Autodesk Inventor part; units mm, degrees
ref_plane "Work Plane1" through (30, 0, 0) normal (0, -0.5, 0.866) x (1, 0, 0)
ref_plane "YZ Plane" through (0, 0, 0) normal (1, 0, 0) x (0, 1, 0)
ref_plane "XZ Plane" through (0, 0, 0) normal (0, 1, 0) x (-1, 0, 0)
sketch "Sketch1" plane through (0, 0, 0) normal (0, 0, 1) x (1, 0, 0)
  line L0 (0.1133, 0) -> (16, 0)
  line L1 (16, 0) -> (16, 3)
  line L2 (16, 3) -> (2, 3)
  line L3 (2, 3) -> (1.3865, 3)
  line L4 (1.3865, 3) -> (0, 3)
  line L5 (0, 3) -> (0, 5.25)
  line L6 (0, 5.25) -> (-3.3, 5.25)
  line L7 (-3.3, 5.25) -> (-3.3, 2.3094)
  line L8 (-3.3, 2.3094) -> (-1.22, 2.3094)
  line L9 (-1.22, 2.3094) -> (0.1133, 0)
  line L10 (-7.16, 0) -> (19.86, 0)
  line L11 (0, -1.05) -> (0, 6.3)
  line L12 (2, 3) -> (0, 3) construction
  dimension "d0" = 14
  dimension "d1" = 0.6135
  dimension "d2" = 3.3
  dimension "d3" = 2.08
  dimension "d4" = 60
  dimension "d5" = 6
  dimension "d6" = 6
  dimension "d7" = 4.6188
  dimension "d8" = 10.5
  dimension "d19" = 16
revolve "Body" add sketch "Sketch1" angle 360 about axis through (0.1133, 0, 0) along (1, 0, 0) contours L9 L11 L4 L3 L2 L1 L0 | L9 L8 L7 L6 L5 L11
sketch "Sketch2" plane through (-3.3, 0, 0) normal (-1, 0, 0) x (0, 0, 1)
  circle A0 centre (0, 0) radius 2.3094
  line L0 (0, -7.35) -> (0, 7.35)
  line L1 (-7.35, 0) -> (7.35, 0)
  line L2 (2.3094, 0) -> (1.1547, -2)
  line L3 (1.1547, -2) -> (-1.1547, -2)
  line L4 (-1.1547, -2) -> (-2.3094, 0)
  line L5 (-2.3094, 0) -> (-1.1547, 2)
  line L6 (-1.1547, 2) -> (1.1547, 2)
  line L7 (1.1547, 2) -> (2.3094, 0)
extrude "Slot" add sketch "Sketch2" against normal up to next contours L7 A0 | A0 L2 | L6 L0 A0 | A0 L0 L3 | L0 L6 A0 | A0 L3 L0 | L4 A0 | A0 L5
fillet "Fillet1" radius 2.5 1 edges at (-3.3, -5.25, 0)
thread "Thread"
chamfer "Chamfer1" distance 0.6135 distance2 0.6135 1 edges at (16, -3, 0) measured on face at (16, -1.1424, 0.935)
fillet "Fillet2" radius 0.25 1 edges at (0, -3, 0)
ref_plane "Work Plane1" through (30, 0, 0) normal (0, -0.5, 0.866) x (1, 0, 0)
equation "\"d0\" = GEL"
equation "\"d1\" = GAL"
equation "\"d2\" = KOH"
equation "\"d3\" = INTI"
equation "\"d5\" = GD"
equation "\"d6\" = BDM"
equation "\"d7\" = 1.1547 * SW"
equation "\"d8\" = KOD"
equation "\"d19\" = NLG"
equation "\"d16\" = RR"
equation "\"d12\" = GEL"
equation "\"d14\" = -0.5 * SPD + 0.5 * GD"
equation "\"d15\" = GUL"
equation "\"d29\" = R"
equation "\"GD\" = NND"
equation "\"NLG\" = 16"
equation "\"GEL\" = 14"
equation "\"KOD\" = 10.5"
equation "\"KOH\" = 3.3"
equation "\"INTI\" = 2.08"
equation "\"GAL\" = 0.61345 * PTC"
equation "\"GUL\" = 0.61345 * PTC"
equation "\"BDM\" = NND"
equation "\"SW\" = 4"
equation "\"RR\" = 2.5"
equation "\"SPD\" = 4.7731"
equation "\"d28\" = R"
equation "\"R\" = 0.25"
equation "\"TOA\" = 30deg"
equation "\"THREADDIA\" = 6"
equation "\"KOD1\" = KOD - 2 * RR"
equation "\"PTC\" = 1"
equation "\"NND\" = 6"
equation "\"E0\" = 1.155 * SW"
equation "\"GD1\" = THREADDIA - 1.2269 * PTC"
properties part number "ANSI B18.3.4M - M6 x 1 x 16, FHSBHCSM" material "Steel, Mild"
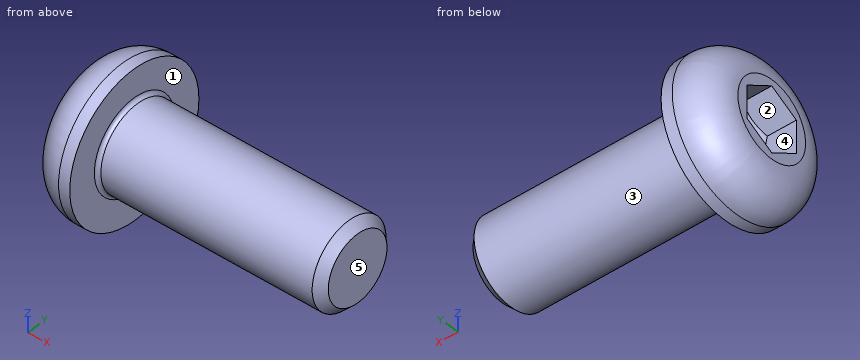
Here's how the part is built. I have some questions about the finished solid (model axes, mm). Face numbers are marked on the shaded views. A direction names the side the tool comes from. Coordinates: 2 decimals unless noted, no trailing zeros. Write each loop counter-clockwise with the first axis right and the second up, starting at its lowest first coordinate (ties: lowest second). Pieces come first, ordered by that corner, then holes.
Item 1: I want a section at A-A on x = 4. Write out the boundary of the cut face in (y, z).
Item 2: I want a section at B-B on x = -0.5. Write out the boundary of the cut face in (y, z).
Item 3: If I drill on line 1 (X direction, y = -1.5, z = -0.5); line 2 (Z direction, x = 11, y = 0); line 3 (X direction, y = -3, z = 1.25), over which ranges is the centre line in solid material (lowest first)?
Item 4: Will these pins go through, and if not, where does the flat tip stop? pin 1 (2.5 mm diameter, centred on x = -2, z = -0.5, fed in from +Y); pin 2 (2 mm diameter, centred on x = 13, z = 3, fed in from -Y); pin 3 (2.5 mm diameter, centred on x = -2.5, z = 0, fed in from -Y); pin 4 (2 mm diameter, centred on x = 8.5, z = 0.5, fed in from -Y).
Item 5: On a 3-axis mill with a long thin cutter (end or side, diameter ignored), from which of +Z, -Z, +X, -X, +Y, -Y can I reach the whole of each face in a straight line? I mean the marked faces 1 and 2. Say none if no direction works.
Item 6: If we mould it in two halves opening along Z, with no side actions, what happens to the marked faces 3, 4 and 5? For each: +Z half, -Z half, draft (parallel to the pull), parting line (faces both ways), or undercut.
Findings below:
1. outline: circle Ø6 at (0, 0)
2. outline: circle Ø10.5 at (0, 0); hole circle Ø2.12 at (0, 0)
3. line 1: x = -0.8 to 16
3. line 2: z = -3 to 3
3. line 3: x = -3.25 to 0
4. pin 1: stops at y = 5.25
4. pin 2: stops at y = -2.24
4. pin 3: stops at y = -5.21
4. pin 4: stops at y = -3
5. face 1: +X
5. face 2: -X
6. face 3: parting line
6. face 4: undercut
6. face 5: draft
